Verification items for this drawing (mm, ordinates from the low corner). A direction names the side the tool comes from. Round coordinates to 2 decimals unless told otherwise and drop trailing zeros. Order: outer loops, then holes, each group sorted by start corner. A loop starts at its lowest first (then second) coordinate and runs counter-clockwise, first axis right, second up. Notation, with made-up numbers: M 80,85 L 112,85 A14 ccw 112,95 Z; hole C 28.25,43 d3. An arc over 180 degrees is marked long. Use CSV: the item, a comma, the result in double quotes. Start each with the question number.
Q1. Sectioned sample at C-C (y = 8.25). Enter the section's corners in (x, z) (1 decimal), and give its area (3 significant figures).
Q2. Scan lines: line 1 (Z direction, x = 1.25, y = 3.5) (1 decimal); line 2 (Z direction, x = 8, y = 8); line 3 (Y direction, x = 5.5, z = 13.5). Record each from-to range of solid material in increasing order.
Q3. Set-up check for the marked faces 1, 2 and 3: record each of +Z, -Z, +X, -X, +Y, -Y from which the full face is reachable in a straight line by a thin tool's end or side.
Q4. Gauge pin test, flat ends, axial feed: pin 1 Ø5 at (x, y) = (9.5, 10) entering from +Z; pin 2 Ø2 at (x, z) = (4, 14.5) entering from -Y; pin 3 Ø6 at (x, z) = (6.5, 26) entering from -Y; pin 4 Ø2 at (x, z) = (2, 17.5) entering from +Y. Record the tip position at first contact, or that the pin passes through.
Q5. Sectioned sample at D-D (x = 10). Enter the section's corners in (y, z) (1 decimal).
Q6. Sectioned sample at A-A (x = 5.25). Enter the section's corners in (y, z) (1 decimal), and give its area (3 significant figures).
Q7. Sectioned sample at B-B (z = 28). Enter the section's corners in (x, y) (3 decimals).
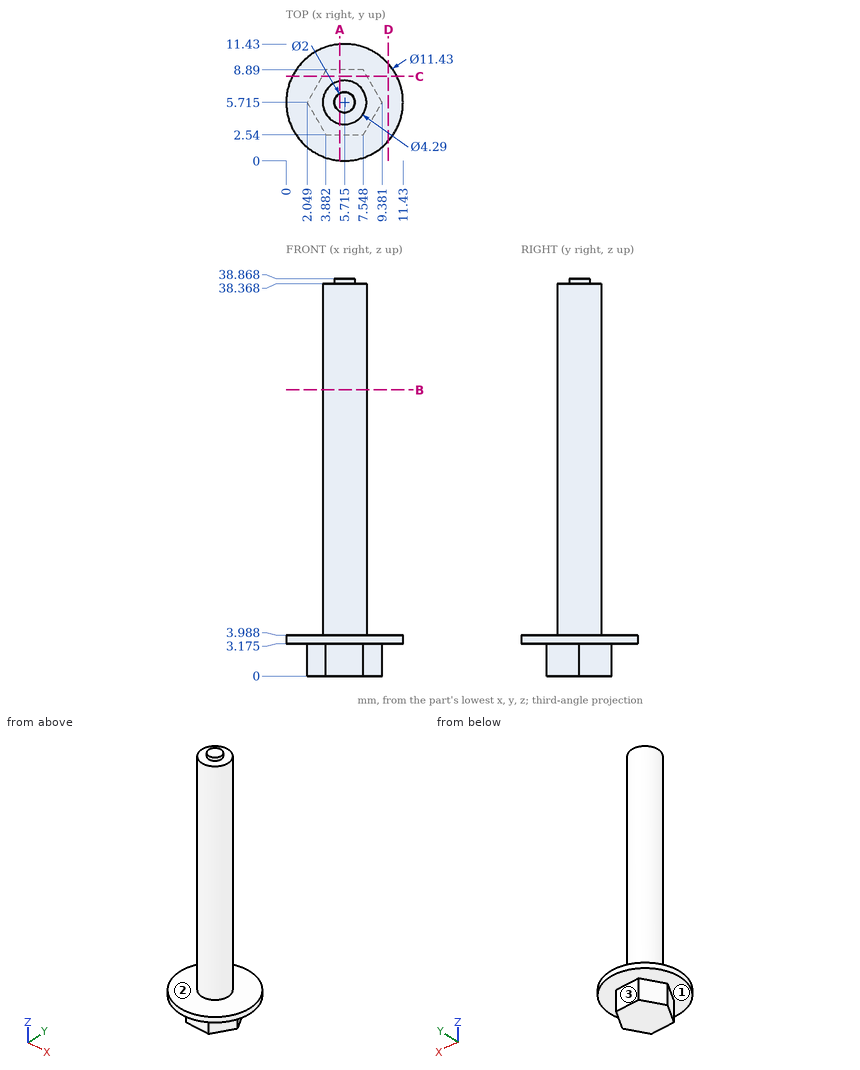
Verdict:
1,outline,"M 0.6,3.2 L 3.5,3.2 L 3.5,0 L 7.9,0 L 7.9,3.2 L 10.8,3.2 L 10.8,4 L 0.6,4 Z"
1,area,"22.3 mm²"
2,line 1,"z = 3.2 to 4"
2,line 2,"z = 0 to 3.99"
2,line 3,"y = 3.58 to 7.85"
3,face 1,"-Z"
3,face 2,"+Z"
3,face 3,"-Z, +X, -X, +Y"
4,pin 1,"stops at z = 3.99"
4,pin 2,"stops at y = 3.69"
4,pin 3,"stops at y = 3.57"
4,pin 4,"passes through"
5,outline,"M 1.9,3.2 L 9.5,3.2 L 9.5,4 L 1.9,4 Z"
6,outline,"M 0,3.2 L 2.5,3.2 L 2.5,0 L 8.9,0 L 8.9,3.2 L 11.4,3.2 L 11.4,4 L 7.8,4 L 7.8,38.4 L 6.6,38.4 L 6.6,38.9 L 4.8,38.9 L 4.8,38.4 L 3.6,38.4 L 3.6,4 L 0,4 Z"
6,area,"174 mm²"
7,outline,"C 5.715,5.715 d4.29"
